Build history of the part. All positions in model axes, mm. Round coordinates to 2 decimals unless told otherwise and drop trailing zeros. Order: outer loops, then holes, each group sorted by start corner. A loop starts at its lowest first (then second) coordinate and runs counter-clockwise, first axis right, second up. Notation, with made-up numbers: (-12.5, -30.75) - (37.5, -30.75) arc R23 cw to (37.5, -1.75) - close; hole circle Ø10 at (-24, 12.5). An arc over 180 degrees is marked (long way). One line per question, with ' | ' between items. Start each with the question number.
from build123d import *

# Parameters (mm, degrees)
SKETCH_1_W          = 20
SKETCH_1_H          = 20
SKETCH_1_W_2        = 17
SKETCH_1_H_2        = 17
EXTRUDE_1_DEPTH     = 487
SKETCH_3_R          = 2
CUT_EXTRUDE_2_DEPTH = 20
SKETCH_4_R          = 2
CUT_EXTRUDE_3_DEPTH = 20


with BuildPart() as part:
    # 草图1 → 凸台-拉伸1 (new body)
    with BuildSketch(Plane.XY):
        Rectangle(SKETCH_1_W, SKETCH_1_H)
        Rectangle(SKETCH_1_W_2, SKETCH_1_H_2, mode=Mode.SUBTRACT)
    extrude(amount=EXTRUDE_1_DEPTH)

    # 草图3 → 切除-拉伸2 (cut)
    with BuildSketch(Plane(origin=(0, 10, 0), x_dir=(1, 0, 0), z_dir=(0, 1, 0))):
        with Locations(Location((0, -10, 0), (0, 0, 270))):
            Circle(SKETCH_3_R)
        with Locations(Location((0, -477, 0), (0, 0, 270))):
            Circle(SKETCH_3_R)
        with Locations(Location((0, -100, 0), (0, 0, 270))):
            Circle(SKETCH_3_R)
        with Locations(Location((0, -387, 0), (0, 0, 270))):
            Circle(SKETCH_3_R)
        with Locations(Location((0, -186.75, 0), (0, 0, 270))):
            Circle(SKETCH_3_R)
        with Locations(Location((0, -300.25, 0), (0, 0, 270))):
            Circle(SKETCH_3_R)
    extrude(amount=-CUT_EXTRUDE_2_DEPTH, mode=Mode.SUBTRACT)

    # 草图4 → 切除-拉伸3 (cut)
    with BuildSketch(Plane(origin=(0, 10, 0), x_dir=(1, 0, 0), z_dir=(0, 1, 0))):
        with Locations(Location((0, -229.5, 0), (0, 0, 270))):
            Circle(SKETCH_4_R)
        with Locations(Location((0, -257.5, 0), (0, 0, 270))):
            Circle(SKETCH_4_R)
    extrude(amount=-CUT_EXTRUDE_3_DEPTH, mode=Mode.SUBTRACT)


solid = part.part
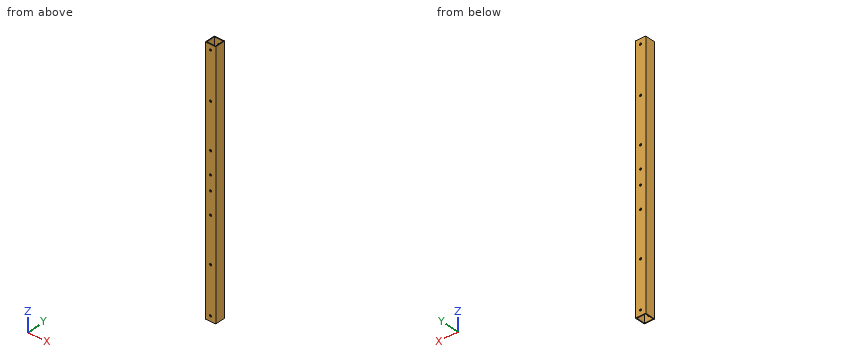
Item 1: Wall check: line 1 along Y through (x, z) = (-6.75, 283); line 2 along X through (y, z) = (9.3, 257.5). Give the ranges that are in metal, low to high. Write a range as [from, to].
Item 2: Slice it at A-A (z = 274). Write the cut outline in (x, y), plus the area to 3 significant figures.
Item 3: Pin check, flat tip, straight feed: pin 1 (3 mm diameter, centred on x = 0, z = 100, fed in from -Y). Stop position of the tip, or through.
Item 4: Slice it at B-B (y = 1). Write the cut outline in (x, z).
A:
1) line 1: [-10, -8.5], [8.5, 10] | line 2: [-10, -2], [2, 10]
2) outline: (-10, -10) - (10, -10) - (10, 10) - (-10, 10) - close; hole (-8.5, -8.5) - (8.5, -8.5) - (8.5, 8.5) - (-8.5, 8.5) - close | area: 111 mm^2
3) pin 1: through
4) outline: (-10, 0) - (-8.5, 0) - (-8.5, 487) - (-10, 487) - close; (8.5, 0) - (10, 0) - (10, 487) - (8.5, 487) - close
